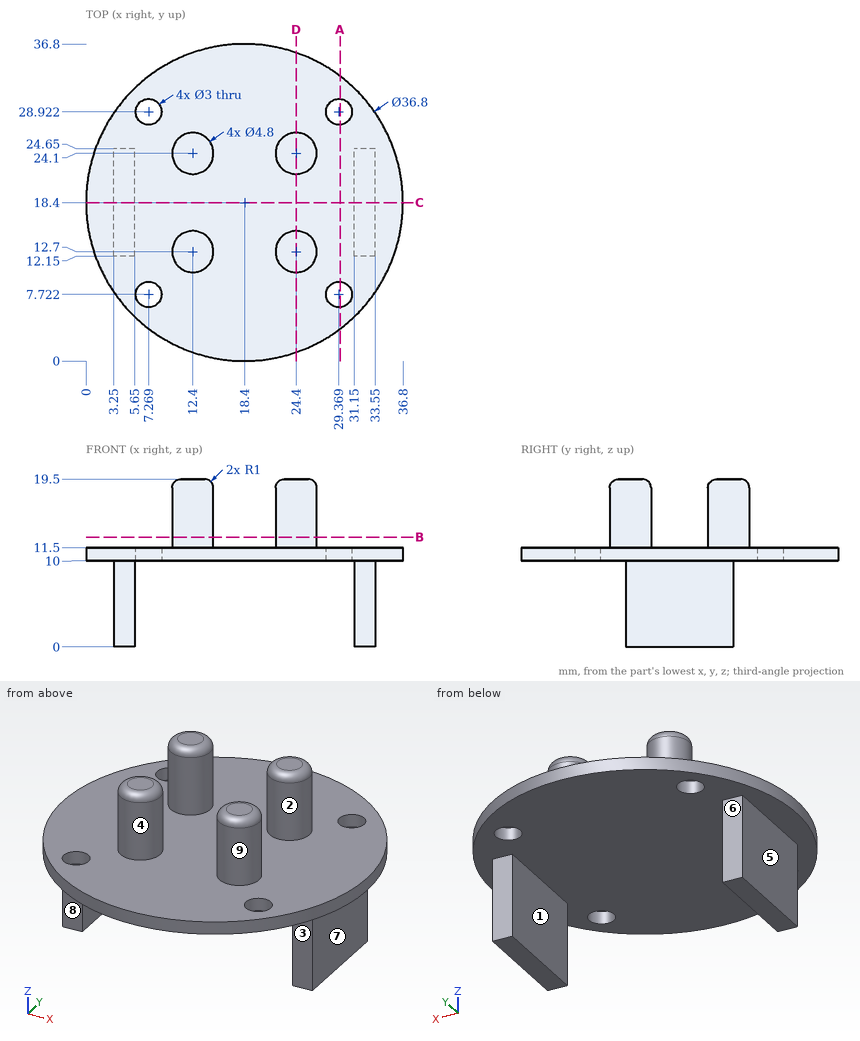
Could you check a few things on this drawing? It's one solid part, dimensions in mm from its lowest x, y, z. A direction names the side the tool comes from. Round coordinates to 2 decimals unless told otherwise and drop trailing zeros. Order: outer loops, then holes, each group sorted by start corner. A loop starts at its lowest first (then second) coordinate and runs counter-clockwise, first axis right, second up. Notation, with made-up numbers: M 63.25,13 L 113.25,13 A22 ccw 113.25,40 Z; hole C 84.5,-32.75 d2. An arc over 180 degrees is marked long. Use a Markdown table: item, result.
1) If I drill on line 1 along X through (y, z) = (24, 7.25); line 2 along Y through (x, z) = (28, 10.5) (1 decimal); line 3 along Y through (x, z) = (24.5, 11.75), over which ranges is the centre line in solid material (lowest first)?
Geometry says:
| item | result |
|---|---|
| line 1 | x = 3.25 to 5.65, 31.15 to 33.55 |
| line 2 | y = 2.7 to 7.1, 8.3 to 28.3, 29.5 to 34.1 |
| line 3 | y = 10.3 to 15.1, 21.7 to 26.5 |
2) Imagine slicing it at B-B (z = 12.75). List the corners of the cut face in (x, y) for me.
Geometry says:
| item | result |
|---|---|
| outline | C 12.4,12.7 d4.8; C 12.4,24.1 d4.8; C 24.4,12.7 d4.8; C 24.4,24.1 d4.8 |
3) On a 3-axis mill with a long thin cutter (end or side, diameter ignored), from which of +Z, -Z, +X, -X, +Y, -Y can I reach the whole of each face in a straight line? I mean the marked faces 5, 6, 7, 8 and 9. Say none if no direction works.
Geometry says:
| item | result |
|---|---|
| face 5 | -Z, -X, +Y, -Y |
| face 6 | -Z, +X, -X, +Y |
| face 7 | -Z, +X, +Y, -Y |
| face 8 | -Z, +X, -X, -Y |
| face 9 | +Z |
4) If we mould it in two halves opening along Y, with no side actions, what happens to the marked faces 1, 2, 3 and 4? For each: +Y half, -Y half, draft (parallel to the pull), parting line (faces both ways), or undercut.
Geometry says:
| item | result |
|---|---|
| face 1 | draft |
| face 2 | undercut |
| face 3 | -Y half |
| face 4 | undercut |
5) Imagine slicing it at A-A (x = 29.5). List the corners of the cut face in (y, z) for me (1 decimal).
Geometry says:
| item | result |
|---|---|
| outline | M 3.7,10 L 6.2,10 L 6.2,11.5 L 3.7,11.5 Z; M 9.2,10 L 27.4,10 L 27.4,11.5 L 9.2,11.5 Z; M 30.4,10 L 33.1,10 L 33.1,11.5 L 30.4,11.5 Z |
6) Imagine slicing it at C-C (y = 18.4). List the corners of the cut face in (x, z) for me, then the cut area to 3 significant figures.
Geometry says:
| item | result |
|---|---|
| outline | M 0,10 L 3.25,10 L 3.25,0 L 5.65,0 L 5.65,10 L 31.15,10 L 31.15,0 L 33.55,0 L 33.55,10 L 36.8,10 L 36.8,11.5 L 0,11.5 Z |
| area | 103 mm² |
7) Imagine slicing it at D-D (x = 24.4). List the corners of the cut face in (y, z) for me.
Geometry says:
| item | result |
|---|---|
| outline | M 1.01,10 L 35.79,10 L 35.79,11.5 L 26.5,11.5 L 26.5,18.5 A1 ccw 25.5,19.5 L 22.7,19.5 A1 ccw 21.7,18.5 L 21.7,11.5 L 15.1,11.5 L 15.1,18.5 A1 ccw 14.1,19.5 L 11.3,19.5 A1 ccw 10.3,18.5 L 10.3,11.5 L 1.01,11.5 Z |
8) I'm going to push flat-ended pins straight in: P1, Ø1.9, axis at x = 32.5, z = 3.5, coming from the -Y side; P2, Ø10, axis at x = 18, z = 10, coming from the -Y side; P3, Ø2.5, axis at x = 29.37, y = 28.92, coming from the +Z side; P4, Ø1, axis at x = 25, y = 26.5, coming from the +Z side. Where does each tip first touch, or does it pass through?
Geometry says:
| item | result |
|---|---|
| P1 | stops at y = 12.15 |
| P2 | stops at y = 0 |
| P3 | passes through |
| P4 | stops at z = 19.32 |
